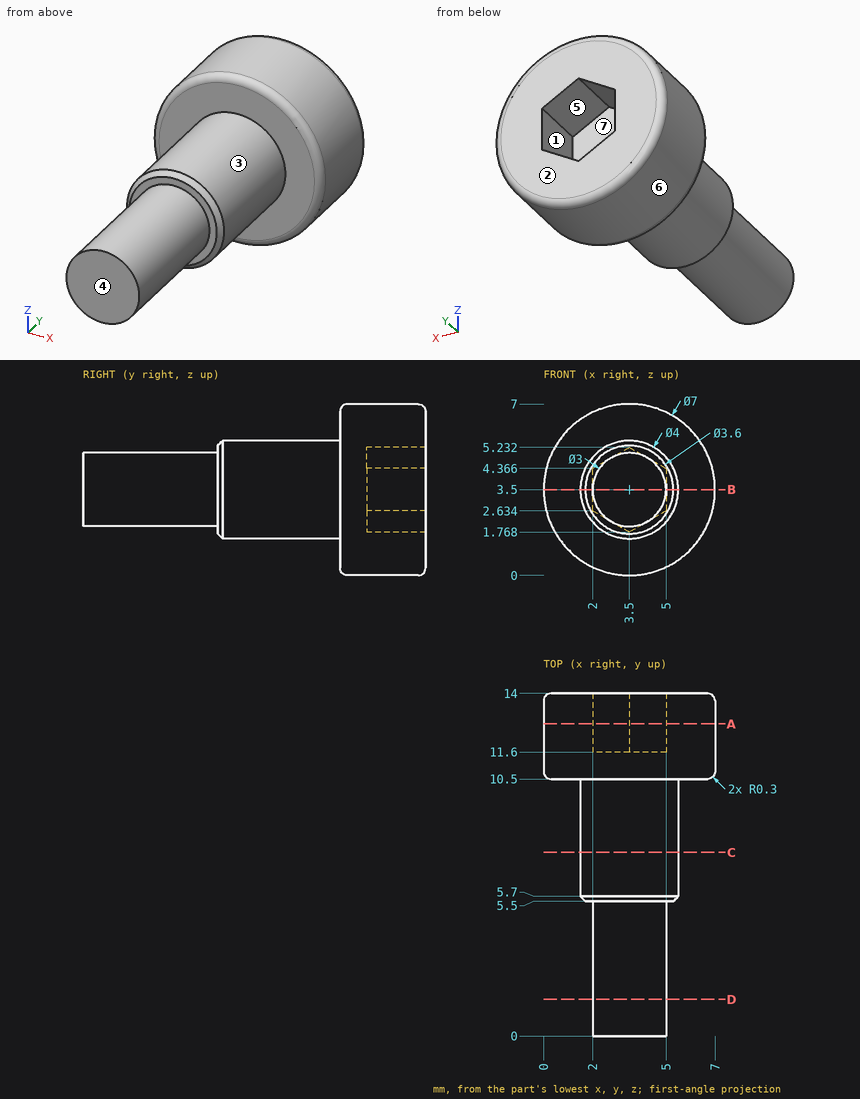
The figure shows three views and two pictorial views of one solid part (mm, origin at its lowest corner). Answer the questions. A direction names the side the tool comes from. Coordinates: 2 decimals unless noted, no trailing zeros. Loops run counter-clockwise (first coordinate to the right, second up) from the corner with the lowest first, then second, coordinate; pieces in that order, holes last.
(1) The part is cut by section B-B (z = 3.5). Determine the outline of the cut face in (x, y), and give its area (3 significant figures).
Solution:
outline: (0, 10.8) arc R0.3 ccw to (0.3, 10.5) - (1.5, 10.5) - (1.5, 5.7) - (1.7, 5.5) - (2, 5.5) - (2, 0) - (5, 0) - (5, 5.5) - (5.3, 5.5) - (5.5, 5.7) - (5.5, 10.5) - (6.7, 10.5) arc R0.3 ccw to (7, 10.8) - (7, 13.7) arc R0.3 ccw to (6.7, 14) - (5, 14) - (5, 11.6) - (2, 11.6) - (2, 14) - (0.3, 14) arc R0.3 ccw to (0, 13.7) - close
area: 53.7 mm2
(2) The mould has two halves that part along X. Classify the marked faces 4, 5, 6 and 7: released by +X, released by -X, zero draft, split by the parting line, or undercut.
Solution:
face 4: zero draft
face 5: undercut
face 6: split by the parting line
face 7: undercut
(3) The part is cut by section D-D (y = 1.5). Determine the outline of the cut face in (x, z), and give its area (3 significant figures).
Solution:
outline: circle Ø3 at (3.5, 3.5)
area: 7.07 mm2
(4) The part is cut by section C-C (y = 7.5). Determine the outline of the cut face in (x, z), and give its area (3 significant figures).
Solution:
outline: circle Ø4 at (3.5, 3.5)
area: 12.6 mm2
(5) Flat-ended cylindrical pins translate along their axes: pin 1 Ø4 at (y, z) = (2, 3) entering from -X; pin 2 Ø2 at (x, y) = (3.5, 3.5) entering from -Z; pin 3 Ø4 at (y, z) = (7, 2) entering from -X. Find the tip coordinate at first contact, or state that the pin passes through.
Solution:
pin 1: stops at x = 2
pin 2: stops at z = 2
pin 3: stops at x = 1.5
(6) The part is cut by section A-A (y = 12.75). Determine the outline of the cut face in (x, z).
Solution:
outline: circle Ø7 at (3.5, 3.5); hole (2, 2.63) - (3.5, 1.77) - (5, 2.63) - (5, 4.37) - (3.5, 5.23) - (2, 4.37) - close
(7) Consider line 1 along Z through (x, y) = (3.5, 4.75); line 2 along Y through (x, z) = (6.5, 2.5); line 3 along Z through (x, y) = (2.75, 12). Determine where each line is inside the solid, lowest interval first.
Solution:
line 1: z = 2 to 5
line 2: y = 10.5 to 14
line 3: z = 0.08 to 2.2, 4.8 to 6.92
(8) A tool of negligible diameter and unlimited length cuts with its end or side. For the marked faces 1, 2 and 3, from which of +Z, -Z, +X, -X, +Y, -Y can it reach the whole face along a straight path? Write none if from no direction.
Solution:
face 1: +Y
face 2: +Z, -Z, +X, -X, +Y
face 3: -Y
